Source: CAD feature listing. Evaluate the final solid. Frame: model axes, mm. A direction names the side the tool comes from. Coordinates: 2 decimals unless noted, no trailing zeros. Order: outer loops, then holes, each group sorted by start corner. A loop starts at its lowest first (then second) coordinate and runs counter-clockwise, first axis right, second up.
```python
from build123d import *

# Parameters (mm, degrees)
SKETCH_1_W          = 8
SKETCH_1_H          = 70
SKETCH_1_R          = 1.5
EXTRUDE_1_DEPTH     = 2.5
SKETCH_4_W          = 70
SKETCH_4_H          = 2.5
EXTRUDE_3_DEPTH     = 12
EXTRUDE_4_DEPTH     = 70
SKETCH_7_R          = 3.1
SKETCH_7_R_2        = 2.1
EXTRUDE_2_DEPTH     = 5
SKETCH_8_W          = 70
SKETCH_8_H          = 2.5
EXTRUDE_5_DEPTH     = 5
CUT_EXTRUDE_1_REACH = 28.076
SKETCH_9_R          = 2.1
CUT_EXTRUDE_2_DEPTH = 10
EXTRUDE_6_REACH     = 29.127
SKETCH_15_W         = 1.5
SKETCH_15_H         = 2
SKETCH_15_W_2       = 2


with BuildPart() as part:
    # 草图1 → 凸台-拉伸1 (new body)
    with BuildSketch(Plane(origin=(0, 0, 0), x_dir=(1, 0, 0), z_dir=(0, 1, 0))):
        Rectangle(SKETCH_1_W, SKETCH_1_H)
        with Locations((0, 30)):
            Circle(SKETCH_1_R, mode=Mode.SUBTRACT)
        with Locations((0, 20)):
            Circle(SKETCH_1_R, mode=Mode.SUBTRACT)
        with Locations((0, -20)):
            Circle(SKETCH_1_R, mode=Mode.SUBTRACT)
        with Locations((0, -30)):
            Circle(SKETCH_1_R, mode=Mode.SUBTRACT)
    extrude(amount=EXTRUDE_1_DEPTH)

    # 草图4 → 凸台-拉伸3 (add)
    with BuildSketch(Plane.ZY.offset(4)):
        with Locations((0, 1.25)):
            Rectangle(SKETCH_4_W, SKETCH_4_H)
    extrude(amount=EXTRUDE_3_DEPTH)

    # 草图6 → 凸台-拉伸4 (add)
    with BuildSketch(Plane.XY.offset(35)):
        with BuildLine():
            Line((-16.855050358, 2.349231552), (-16, 0))
            Line((-16, 0), (-16, 2.5))
            ThreePointArc((-16, 2.5), (-16.434120444, 2.462019383), (-16.855050358, 2.349231552))
        make_face()
    extrude(amount=-EXTRUDE_4_DEPTH)

    # 草图7 → 拉伸-薄壁2 (add)
    with BuildSketch(Plane(origin=(-14.128355545, -5.142300877, 0), x_dir=(0, 0, 1), z_dir=(-0.939692621, -0.342020143, 0))):
        with Locations((30, 9.472322293)):
            Circle(SKETCH_7_R)
        with Locations((30, 9.472322293)):
            Circle(SKETCH_7_R_2, mode=Mode.SUBTRACT)
        with Locations((-30, 9.472322293)):
            Circle(SKETCH_7_R)
        with Locations((-30, 9.472322293)):
            Circle(SKETCH_7_R_2, mode=Mode.SUBTRACT)
    extrude(amount=EXTRUDE_2_DEPTH)

    # 草图8 → 凸台-拉伸5 (add)
    with BuildSketch(Plane(origin=(-14.128355545, -5.142300877, 0), x_dir=(0, 0, 1), z_dir=(-0.939692621, -0.342020143, 0))):
        with Locations((0, 6.722322293)):
            Rectangle(SKETCH_8_W, SKETCH_8_H)
    extrude(amount=EXTRUDE_5_DEPTH)

    # 草图9 → 切除-拉伸1 (cut, up to next)
    with BuildSketch(Plane(origin=(-18.826818649, -6.852401594, 0), x_dir=(0, 0, 1), z_dir=(-0.939692621, -0.342020143, 0)), mode=Mode.PRIVATE) as cut_extrude_1_sk1:
        with Locations((-30, 9.472322293)):
            Circle(SKETCH_9_R)
    cut_extrude_1_tool1 = extrude(cut_extrude_1_sk1.sketch, amount=-CUT_EXTRUDE_1_REACH, mode=Mode.PRIVATE) & part.part
    add(cut_extrude_1_tool1.solids().sort_by_distance((-22.066544, 2.04867, -30))[0], mode=Mode.SUBTRACT)
    # 草图9 → 切除-拉伸1 (cut, up to next)
    with BuildSketch(Plane(origin=(-18.826818649, -6.852401594, 0), x_dir=(0, 0, 1), z_dir=(-0.939692621, -0.342020143, 0)), mode=Mode.PRIVATE) as cut_extrude_1_sk2:
        with Locations((30, 9.472322293)):
            Circle(SKETCH_9_R)
    cut_extrude_1_tool2 = extrude(cut_extrude_1_sk2.sketch, amount=-CUT_EXTRUDE_1_REACH, mode=Mode.PRIVATE) & part.part
    add(cut_extrude_1_tool2.solids().sort_by_distance((-22.066544, 2.04867, 30))[0], mode=Mode.SUBTRACT)

    # 草图11 → 切除-拉伸2 (cut)
    with BuildSketch(Plane(origin=(0, 2.5, 0), x_dir=(1, 0, 0), z_dir=(0, 1, 0))):
        with BuildLine():
            Line((1.500000061, 28.40000046), (-10.499999939, 28.4))
            ThreePointArc((-10.499999939, 28.4), (-12.1, 29.999999939), (-10.500000061, 31.6))
            Line((-10.500000061, 31.6), (1.499999939, 31.60000046))
            ThreePointArc((1.499999939, 31.60000046), (3.1, 30.000000521), (1.500000061, 28.40000046))
        make_face()
        with BuildLine():
            Line((1.500000061, -31.59999977), (-10.499999939, -31.60000023))
            ThreePointArc((-10.499999939, -31.60000023), (-12.1, -30.000000291), (-10.500000061, -28.40000023))
            Line((-10.500000061, -28.40000023), (1.499999939, -28.39999977))
            ThreePointArc((1.499999939, -28.39999977), (3.1, -29.999999709), (1.500000061, -31.59999977))
        make_face()
    extrude(amount=-CUT_EXTRUDE_2_DEPTH, mode=Mode.SUBTRACT)

    # 凸台-拉伸6: up to this face of the body (flat: up to its plane)
    extrude_6_end = Plane(part.part.faces().sort_by_distance((-21.270490347, -0.138468784, 0))[0])
    # 草图15 → 凸台-拉伸6 (add, up to the picked face)
    with BuildSketch(Plane(origin=(4, 0, 0), x_dir=(0, 0, -1), z_dir=(1, 0, 0)), mode=Mode.PRIVATE) as extrude_6_sk1:
        with Locations((-34.25, -1)):
            Rectangle(SKETCH_15_W, SKETCH_15_H)
    extrude_6_tool1 = split(extrude(extrude_6_sk1.sketch, amount=-EXTRUDE_6_REACH, mode=Mode.PRIVATE), bisect_by=extrude_6_end, keep=Keep.BOTH, mode=Mode.PRIVATE)
    add(extrude_6_tool1.solids().sort_by_distance((4, -1, 34.25))[0])
    # 草图15 → 凸台-拉伸6 (add, up to the picked face)
    with BuildSketch(Plane(origin=(4, 0, 0), x_dir=(0, 0, -1), z_dir=(1, 0, 0)), mode=Mode.PRIVATE) as extrude_6_sk2:
        with Locations((-24.5, -1)):
            Rectangle(SKETCH_15_W_2, SKETCH_15_H)
    extrude_6_tool2 = split(extrude(extrude_6_sk2.sketch, amount=-EXTRUDE_6_REACH, mode=Mode.PRIVATE), bisect_by=extrude_6_end, keep=Keep.BOTH, mode=Mode.PRIVATE)
    add(extrude_6_tool2.solids().sort_by_distance((4, -1, 24.5))[0])
    # 草图15 → 凸台-拉伸6 (add, up to the picked face)
    with BuildSketch(Plane(origin=(4, 0, 0), x_dir=(0, 0, -1), z_dir=(1, 0, 0)), mode=Mode.PRIVATE) as extrude_6_sk3:
        with Locations((-13.5, -1)):
            Rectangle(SKETCH_15_W_2, SKETCH_15_H)
    extrude_6_tool3 = split(extrude(extrude_6_sk3.sketch, amount=-EXTRUDE_6_REACH, mode=Mode.PRIVATE), bisect_by=extrude_6_end, keep=Keep.BOTH, mode=Mode.PRIVATE)
    add(extrude_6_tool3.solids().sort_by_distance((4, -1, 13.5))[0])
    # 草图15 → 凸台-拉伸6 (add, up to the picked face)
    with BuildSketch(Plane(origin=(4, 0, 0), x_dir=(0, 0, -1), z_dir=(1, 0, 0)), mode=Mode.PRIVATE) as extrude_6_sk4:
        with Locations((-5.5, -1)):
            Rectangle(SKETCH_15_W_2, SKETCH_15_H)
    extrude_6_tool4 = split(extrude(extrude_6_sk4.sketch, amount=-EXTRUDE_6_REACH, mode=Mode.PRIVATE), bisect_by=extrude_6_end, keep=Keep.BOTH, mode=Mode.PRIVATE)
    add(extrude_6_tool4.solids().sort_by_distance((4, -1, 5.5))[0])
    # 草图15 → 凸台-拉伸6 (add, up to the picked face)
    with BuildSketch(Plane(origin=(4, 0, 0), x_dir=(0, 0, -1), z_dir=(1, 0, 0)), mode=Mode.PRIVATE) as extrude_6_sk5:
        with Locations((5.5, -1)):
            Rectangle(SKETCH_15_W_2, SKETCH_15_H)
    extrude_6_tool5 = split(extrude(extrude_6_sk5.sketch, amount=-EXTRUDE_6_REACH, mode=Mode.PRIVATE), bisect_by=extrude_6_end, keep=Keep.BOTH, mode=Mode.PRIVATE)
    add(extrude_6_tool5.solids().sort_by_distance((4, -1, -5.5))[0])
    # 草图15 → 凸台-拉伸6 (add, up to the picked face)
    with BuildSketch(Plane(origin=(4, 0, 0), x_dir=(0, 0, -1), z_dir=(1, 0, 0)), mode=Mode.PRIVATE) as extrude_6_sk6:
        with Locations((13.5, -1)):
            Rectangle(SKETCH_15_W_2, SKETCH_15_H)
    extrude_6_tool6 = split(extrude(extrude_6_sk6.sketch, amount=-EXTRUDE_6_REACH, mode=Mode.PRIVATE), bisect_by=extrude_6_end, keep=Keep.BOTH, mode=Mode.PRIVATE)
    add(extrude_6_tool6.solids().sort_by_distance((4, -1, -13.5))[0])
    # 草图15 → 凸台-拉伸6 (add, up to the picked face)
    with BuildSketch(Plane(origin=(4, 0, 0), x_dir=(0, 0, -1), z_dir=(1, 0, 0)), mode=Mode.PRIVATE) as extrude_6_sk7:
        with Locations((34.25, -1)):
            Rectangle(SKETCH_15_W, SKETCH_15_H)
    extrude_6_tool7 = split(extrude(extrude_6_sk7.sketch, amount=-EXTRUDE_6_REACH, mode=Mode.PRIVATE), bisect_by=extrude_6_end, keep=Keep.BOTH, mode=Mode.PRIVATE)
    add(extrude_6_tool7.solids().sort_by_distance((4, -1, -34.25))[0])
    # 草图15 → 凸台-拉伸6 (add, up to the picked face)
    with BuildSketch(Plane(origin=(4, 0, 0), x_dir=(0, 0, -1), z_dir=(1, 0, 0)), mode=Mode.PRIVATE) as extrude_6_sk8:
        with Locations((24.5, -1)):
            Rectangle(SKETCH_15_W_2, SKETCH_15_H)
    extrude_6_tool8 = split(extrude(extrude_6_sk8.sketch, amount=-EXTRUDE_6_REACH, mode=Mode.PRIVATE), bisect_by=extrude_6_end, keep=Keep.BOTH, mode=Mode.PRIVATE)
    add(extrude_6_tool8.solids().sort_by_distance((4, -1, -24.5))[0])


solid = part.part
```
Q1. Section query A-A on z = -20. Output: boundary loops of the cut face in (x, y).
Solutions:
outline: (-21.55, 0.64) - (-20.7, -1.71) - (-16, 0) - (-1.5, 0) - (-1.5, 2.5) - (-16, 2.5) arc R2.5 ccw to (-16.86, 2.35) - close; (1.5, 0) - (4, 0) - (4, 2.5) - (1.5, 2.5) - close
Q2. Pin query (flat end, axial travel): P1, Ø10, axis at x = -14, z = 16.5, coming from the +Y side; P2, Ø6.5, axis at x = -1.5, z = -30, coming from the -Y side; P3, Ø2, axis at y = 1, z = -19.5, coming from the -X side; P4, Ø12, axis at x = -6, z = 9, coming from the -Y side. Return the tip coordinate at first contact, or that it passes through.
Solutions:
P1: stops at y = 2.5
P2: stops at y = 0
P3: stops at x = -21.55
P4: stops at y = -2
Q3. Section query C-C on z = 30. Output: boundary loops of the cut face in (x, y), plus the area to 3 significant figures.
Solutions:
outline: (-23.13, 4.96) - (-22.78, 4.02) - (-18.09, 5.73) - (-18.43, 6.67) - close; (-21.35, 0.08) - (-20.7, -1.71) - (-16, 0) - (-12.1, 0) - (-12.1, 2.5) - (-14.69, 2.5) - close; (3.1, 0) - (4, 0) - (4, 2.5) - (3.1, 2.5) - close
area: 26.8 mm2
Q4. Pull-direction query (X, two-part tool) for faces 4 (the cylindrical face through (-12.1, 1.3, -30)), 5 (the flat face through (-18.316, -0.843, -29.556)), 6 (the flat face through (-6, 0, 28)), 7 (the flat face through (-4, 1, 31.6)); classes: pulls with the +X half, pulls with the -X half, needs draft (parallel to the pull), parting line crosses it, or undercut.
Solutions:
face 4: undercut
face 5: pulls with the +X half
face 6: needs draft
face 7: undercut
Q5. Section query B-B on x = -5.5. Give the number of separate pieces and of enclosed holes in the cut face, plus the area to 3 significant figures.
Solutions:
separate pieces: 3
enclosed holes: 0
area: 189 mm2
Q6. Material intervals for line 1 along Z through (x, y) = (-3.75, 2); line 2 along Z through (x, y) = (0, 1.9); line 3 along Z through (x, y) = (2.5, 1.5), sorted ascending.
Solutions:
line 1: z = -35 to -31.6, -28.4 to 28.4, 31.6 to 35
line 2: z = -35 to -31.6, -28.4 to -21.5, -18.5 to 18.5, 21.5 to 28.4, 31.6 to 35
line 3: z = -35 to -31.25, -28.75 to 28.75, 31.25 to 35
Q7. Set-up query: faces 1 (the flat face through (-9, 0, -35)), 2 (the flat face through (-18.316, -0.843, 18.937)), 3 (the cylindrical face through (3.1, 1.3, -30)). Return all of +Z, -Z, +X, -X, +Y, -Y with unobstructed straight access to the full face (end or side cutting, diameter ignored); none if empty.
Solutions:
face 1: -Z, +X, -X, +Y, -Y
face 2: +X, -Y
face 3: +Y, -Y
